Verification items for the finished model (mm, model axes). A direction names the side the tool comes from. Round coordinates to 2 decimals unless told otherwise and drop trailing zeros. Write each loop counter-clockwise with the first axis right and the second up, starting at its lowest first coordinate (ties: lowest second). Pieces come first, ordered by that corner, then holes. Notation, with made-up numbers: (33, 61.25) -> (45, 61.25) arc R29 cw to (45, 82.25) -> close; hole circle Ø6 at (44.25, -30). An arc over 180 degrees is marked (long way). Use CSV: the item, a comma, the result in double quotes.
Autodesk Inventor part; units mm, degrees
ref_plane "YZ Plane" through (0, 0, 0) normal (1, 0, 0) x (0, 1, 0)
ref_plane "XZ Plane" through (0, 0, 0) normal (0, 1, 0) x (-1, 0, 0)
ref_plane "XY Plane" through (0, 0, 0) normal (0, 0, 1) x (1, 0, 0)
sketch "スケッチ1" plane through (0, 0, 0) normal (0, 0, 1) x (1, 0, 0)
  line L0 (-39, -16) -> (-39, 16)
  line L1 (39, 16) -> (39, -16)
  line L2 (39, -16) -> (-39, 16) construction
  line L3 (-39, -16) -> (39, 16) construction
  line L4 (0, 0) -> (0, 16) construction
  line L5 (0, 0) -> (-39, 0) construction
  line L6 (-39, 16) -> (-24, 16)
  line L7 (-24, 16) -> (-24, -16) construction
  line L8 (-31.5, 16) -> (-31.5, -16) construction
  line L9 (-24, 0) -> (-39, 0) construction
  circle A0 centre (-31.5, 6) radius 1.6
  circle A1 centre (-31.5, -6) radius 1.6
  line L10 (24, 16) -> (24, -16) construction
  line L11 (31.5, 16) -> (31.5, -16) construction
  line L12 (24, 0) -> (39, 0) construction
  circle A2 centre (31.5, 6) radius 1.6
  circle A3 centre (31.5, -6) radius 1.6
  line L13 (-39, 16) -> (-24, 16)
  line L14 (24, 16) -> (39, 16)
  line L15 (39, -16) -> (24, -16)
  line L16 (-24, -16) -> (-39, -16)
  circle A4 centre (0, 0) radius 13.75
  circle A5 centre (0, 13.75) radius 1.6
  circle A6 centre (0, -13.75) radius 1.6
  arc A7 (24, 16) -> (-24, 16) centre (0, -105.3782) ccw
  arc A8 (-24, -16) -> (24, -16) centre (0, 105.3782) ccw
  dimension "d5" = 78
  dimension "d6" = 32
  dimension "d7" = 15
  dimension "d8" = 3.2
  dimension "d9" = 6
  dimension "d44" = 27.5
  dimension "d45" = 3.2
  dimension "d46" = 3.2
  dimension "d47" = 3
  dimension "d48" = 3
extrude "押し出し2" add sketch "スケッチ1" along normal blind 3 contours L0 L6 A7 L14 L1 L15 A8 L16 | A4 A6 A5 | A5 A4 | A4 A5 | A6 A4 | A4 A6
sketch "スケッチ4" plane through (0, 0, 0) normal (0, 0, -1) x (-1, 0, 0)
  circle A0 centre (-31.5, 6) radius 1.6
  circle A1 centre (-31.5, -6) radius 1.6
  circle A2 centre (31.5, -6) radius 1.6
  circle A3 centre (31.5, 6) radius 1.6
  line L0 (24, 16) -> (39, 16)
  line L1 (-39, 16) -> (-24, 16)
  line L2 (-39, -16) -> (-39, 16)
  line L3 (-24, -16) -> (-39, -16)
  line L4 (39, -16) -> (24, -16)
  line L5 (39, 16) -> (39, -16)
  line L6 (-39, 0) -> (39, 0) construction
  line L7 (0, 36) -> (0, -36) construction
  circle A4 centre (0, 0) radius 10.25
  circle A5 centre (0, 0) radius 13.75 construction
  circle A6 centre (0, 13.75) radius 1.6
  circle A7 centre (0, 0) radius 13.75 construction
  circle A8 centre (-9.7227, 9.7227) radius 1.6
  circle A9 centre (0, 0) radius 13.75 construction
  circle A10 centre (-13.75, 0) radius 1.6
  circle A11 centre (0, 0) radius 13.75 construction
  circle A12 centre (-9.7227, -9.7227) radius 1.6
  circle A13 centre (0, 0) radius 13.75 construction
  circle A14 centre (0, -13.75) radius 1.6
  circle A15 centre (0, 0) radius 13.75 construction
  circle A16 centre (9.7227, -9.7227) radius 1.6
  circle A17 centre (0, 0) radius 13.75 construction
  circle A18 centre (13.75, 0) radius 1.6
  circle A19 centre (0, 0) radius 13.75 construction
  circle A20 centre (9.7227, 9.7227) radius 1.6
  arc A21 (24, 16) -> (-24, 16) centre (0, -105.3782) ccw
  arc A22 (-24, -16) -> (24, -16) centre (0, 105.3782) ccw
  dimension "d17" = 27.5
  dimension "d16" = 20.5
  dimension "d18" = 3.2
  dimension "d21" = 360
extrude "押し出し4" cut sketch "スケッチ4" against normal through all contours A4 | A6 | A8 | A10 | A12 | A14 | A16 | A18 | A20
properties part number "サーボ支え板B_アルミ(A2017)_t3" material "アルミニウム 6061"
Q1. Mould release check, pull along X, two halves, no side actions. Record for faces 4 (the cylindrical face through (0.34, -18.35, 1.48)), 5 (the cylindrical face through (15.35, 0.07, 1.48)), 6 (the flat face through (31, 16, 1)), 7 (the flat face through (39, 0, 1)): released by +X, released by -X, zero draft, split by the parting line, or undercut.
Filled in:
face 4,"split by the parting line"
face 5,"undercut"
face 6,"zero draft"
face 7,"released by +X"
Q2. Section check A-A (y = 13.75). Record the cut outline in (x, z), plus the area to 3 significant figures.
Filled in:
outline,"(-39, 0) -> (-1.6, 0) -> (-1.6, 3) -> (-39, 3) -> close; (1.6, 0) -> (39, 0) -> (39, 3) -> (1.6, 3) -> close"
area,"224 mm²"
Q3. Section check B-B (x = 13.75). Record the cut outline in (y, z).
Filled in:
outline,"(-17.58, 0) -> (-1.6, 0) -> (-1.6, 3) -> (-17.58, 3) -> close; (1.6, 0) -> (17.58, 0) -> (17.58, 3) -> (1.6, 3) -> close"
Q4. Material ranges on L1, parallel to Y at x = 31.5, z = 1.1; L2, parallel to X at y = -11, z = 0.7; L3, parallel to Y at x = 8.5, z = 1.5, recorded low to high.
Filled in:
L1,"-16 to -7.6, -4.4 to 4.4, 7.6 to 16"
L2,"-39 to -10.69, -8.76 to 8.76, 10.69 to 39"
L3,"-18.06 to -10.75, -8.69 to -5.73, 5.73 to 8.69, 10.75 to 18.06"
Q5. Section check D-D (z = 1.1). State how many separate pieces and enclosed holes the cut face has, plus the area to 3 significant figures.
Filled in:
separate pieces,"1"
enclosed holes,"13"
area,"2,220 mm²"
Q6. Section check C-C (x = 0). Record the cut outline in (y, z), plus the area to 3 significant figures.
Filled in:
outline,"(-18.35, 0) -> (-15.35, 0) -> (-15.35, 3) -> (-18.35, 3) -> close; (-12.15, 0) -> (-10.25, 0) -> (-10.25, 3) -> (-12.15, 3) -> close; (10.25, 0) -> (12.15, 0) -> (12.15, 3) -> (10.25, 3) -> close; (15.35, 0) -> (18.35, 0) -> (18.35, 3) -> (15.35, 3) -> close"
area,"29.4 mm²"
Q7. Access from +Z, -Z, +X, -X, +Y, -Y to the whole of each face (thin tool, end or side, straight path). Record for faces 1 (the flat face through (-32, 16, 1)), 2 (the flat face through (32, -16, 1)), 3 (the flat face through (8, -8, 3)).
Filled in:
face 1,"+Z, -Z, -X, +Y"
face 2,"+Z, -Z, +X, -Y"
face 3,"+Z, +X, -X, +Y, -Y"
Q8. Go/stop test with flat-tipped pins: P1, Ø12, axis at x = -21.5, y = -8.5, coming from the -Z side; P2, Ø1.5, axis at x = 32.5, z = 1.5, coming from the +Y side; P3, Ø1, axis at x = -11.5, z = 2, coming from the -Y side; P4, Ø0.9, axis at x = 31.5, z = 2, coming from the -Y side. Record where each tip stops, or that it passes through.
Filled in:
P1,"z = 0"
P2,"y = 16"
P3,"y = -17.86"
P4,"y = -16"
